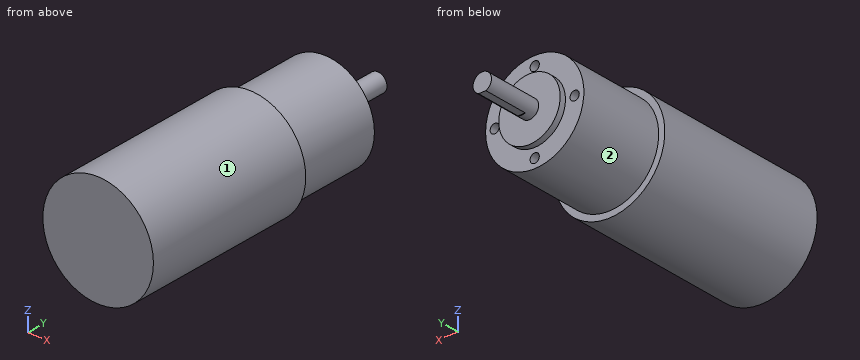
```python
from build123d import *

# Parameters (mm, degrees)
ESQUISSE1_R                  = 18
BOSS_EXTRU_1_DEPTH           = 86.5
ESQUISSE2_R                  = 10
BOSS_EXTRU_2_DEPTH           = 2
ESQUISSE3_R                  = 3
BOSS_EXTRU_3_DEPTH           = 18
ENL_V_MAT_EXTRU_1_DEPTH      = 15
ESQUISSE6_R                  = 1.5
ENL_V_MAT_EXTRU_2_DEPTH      = 10
R_P_TITION_CIRCULAIRE1_COUNT = 4
ESQUISSE7_R                  = 18
ESQUISSE7_R_2                = 16
ENL_V_MAT_EXTRU_3_DEPTH      = 28.5


with BuildPart() as part:
    # Esquisse1 → Boss.-Extru.1 (new body)
    with BuildSketch(Plane(origin=(0, 0, 0), x_dir=(1, 0, 0), z_dir=(0, 1, 0))):
        Circle(ESQUISSE1_R)
    extrude(amount=BOSS_EXTRU_1_DEPTH)

    # Esquisse2 → Boss.-Extru.2 (add)
    with BuildSketch(Plane(origin=(0, 86.5, 0), x_dir=(1, 0, 0), z_dir=(0, 1, 0))):
        Circle(ESQUISSE2_R)
    extrude(amount=BOSS_EXTRU_2_DEPTH)

    # Esquisse3 → Boss.-Extru.3 (add)
    with BuildSketch(Plane(origin=(0, 88.5, 0), x_dir=(1, 0, 0), z_dir=(0, 1, 0))):
        Circle(ESQUISSE3_R)
    extrude(amount=BOSS_EXTRU_3_DEPTH)

    # Esquisse4 → Enl_v. mat.-Extru.1 (cut)
    with BuildSketch(Plane(origin=(0, 106.5, 0), x_dir=(1, 0, 0), z_dir=(0, 1, 0))):
        Polygon((-67.737881949, 2.75), (-1.198957881, 2.75), (1.198957881, 2.75), (67.737881949, 2.75), (67.737881949, 135.827848137), (-67.737881949, 135.827848137), align=None)
    extrude(amount=-ENL_V_MAT_EXTRU_1_DEPTH, mode=Mode.SUBTRACT)

    # Esquisse6 → Enl_v. mat.-Extru.2 (cut)
    with BuildSketch(Plane(origin=(0, 86.5, 0), x_dir=(1, 0, 0), z_dir=(0, 1, 0))):
        with Locations((13, 0)):
            Circle(ESQUISSE6_R)
    enl_v_mat_extru_2 = extrude(amount=-ENL_V_MAT_EXTRU_2_DEPTH, mode=Mode.SUBTRACT)

    # R_p_tition circulaire1: Enl_v. mat.-Extru.2 ×4 about axis
    r_p_tition_circulaire1_axis = Axis((0, 0, 0), (0, 1, 0))
    for i in range(1, R_P_TITION_CIRCULAIRE1_COUNT):
        add(enl_v_mat_extru_2.rotate(r_p_tition_circulaire1_axis, i * 360 / R_P_TITION_CIRCULAIRE1_COUNT), mode=Mode.SUBTRACT)

    # Esquisse7 → Enl_v. mat.-Extru.3 (cut)
    with BuildSketch(Plane(origin=(0, 86.5, 0), x_dir=(1, 0, 0), z_dir=(0, 1, 0))):
        Circle(ESQUISSE7_R)
        Circle(ESQUISSE7_R_2, mode=Mode.SUBTRACT)
    extrude(amount=-ENL_V_MAT_EXTRU_3_DEPTH, mode=Mode.SUBTRACT)


solid = part.part
```
Geometry: final body of the model. Coordinates: model frame, mm. Face numbers are marked on the shaded views. A direction names the side the tool comes from. Coordinates: 2 decimals unless noted, no trailing zeros. Write each loop counter-clockwise with the first axis right and the second up, starting at its lowest first coordinate (ties: lowest second). Pieces come first, ordered by that corner, then holes. Notation, with made-up numbers: M 89.5,-1.75 L 125.5,-1.75 A23 ccw 125.5,14.25 Z; hole C 8.25,16 d5. An arc over 180 degrees is marked long. Use CSV: the item, a comma, the result in double quotes. Start each with the question number.
1. Cut plane D-D on z = 13. Return the cut outline in (x, y), plus the area to 3 significant figures.
2. Ray query, probe 1 along Y at (x, z) = (2, -12); probe 2 along Y at (x, z) = (-7.5, 4.5); probe 3 along Z at (x, y) = (13, 78). Return the intervals inside material, ascending.
3. Cut plane B-B on x = -8.5. Return the cut outline in (y, z).
4. Reachability of the marked faces 1 and 2 from +Z, -Z, +X, -X, +Y, -Y: full face, straight path, thin tool, end or side. Return the list, or none.
5. Cut plane C-C on y = 19. Return the cut outline in (x, z).
6. Cut plane A-A on z = 0. Return the cut outline in (x, y).
7. First-contact query: P1, Ø8, axis at y = 20, z = 5, coming from the -X side; P2, Ø2.5, axis at x = -13, z = -0.5, coming from the +Y side; P3, Ø2.5, axis at x = 0, z = 13, coming from the -Y side; P4, Ø12, axis at y = 59.5, z = 8.5, coming from the -X side. Flat tips, straight axial feed; report the tip coordinate or a pass-through.
Entries:
1,outline,"M -12.45,0 L 12.45,0 L 12.45,58 L 9.33,58 L 9.33,86.5 L 1.5,86.5 L 1.5,76.5 L -1.5,76.5 L -1.5,86.5 L -9.33,86.5 L -9.33,58 L -12.45,58 Z"
1,area,"1,950 mm²"
2,probe 1,"0 to 86.5"
2,probe 2,"0 to 88.5"
2,probe 3,"-9.33 to -1.5, 1.5 to 9.33"
3,outline,"M 0,-15.87 L 58,-15.87 L 58,-13.56 L 86.5,-13.56 L 86.5,-5.27 L 88.5,-5.27 L 88.5,5.27 L 86.5,5.27 L 86.5,13.56 L 58,13.56 L 58,15.87 L 0,15.87 Z"
4,face 1,"+Y, -Y"
4,face 2,"+Y"
5,outline,"C 0,0 d36"
6,outline,"M -18,0 L 18,0 L 18,58 L 16,58 L 16,86.5 L 14.5,86.5 L 14.5,76.5 L 11.5,76.5 L 11.5,86.5 L 10,86.5 L 10,88.5 L 3,88.5 L 3,106.5 L -3,106.5 L -3,88.5 L -10,88.5 L -10,86.5 L -11.5,86.5 L -11.5,76.5 L -14.5,76.5 L -14.5,86.5 L -16,86.5 L -16,58 L -18,58 Z"
7,P1,"x = -17.97"
7,P2,"y = 86.5"
7,P3,"y = 0"
7,P4,"x = -17.8"
